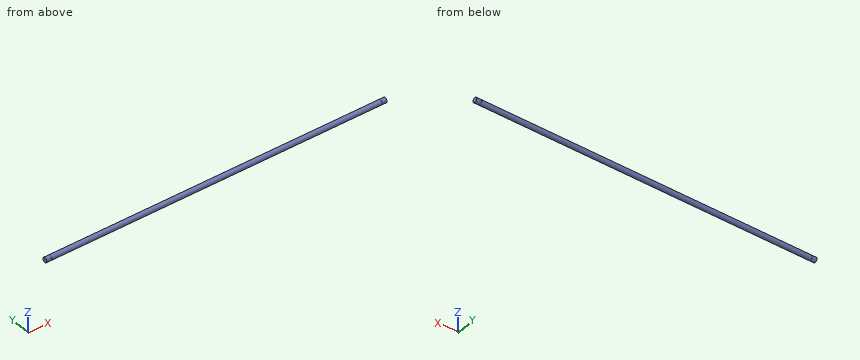
```python
from build123d import *

# Parameters (mm, degrees)
F0_R     = 5
F1_DEPTH = 350
F2_W     = 1.1
F2_H     = 1


with BuildPart() as f1:
    # F0 (on Right) → F1 (new body, symmetric)
    with BuildSketch(Plane.YZ):
        Circle(F0_R)
    extrude(amount=F1_DEPTH, both=True)

    # F2 (on Front) → F3 (revolve, cut)
    with BuildSketch(Plane.XZ):
        with Locations((340.05, 5.3)):
            Rectangle(F2_W, F2_H)
        with Locations((-340.05, 5.3)):
            Rectangle(F2_W, F2_H)
    revolve(axis=Axis((186.2977445126, 0, 0), (1, 0, 0)), mode=Mode.SUBTRACT)


solid = f1.part
```
Design review of the part built by this model. Coordinates are the model's own, in mm. Coordinates: 2 decimals unless noted, no trailing zeros. Write each loop counter-clockwise with the first axis right and the second up, starting at its lowest first coordinate (ties: lowest second). Pieces come first, ordered by that corner, then holes.
1) To check wall thickness, follow L1, parallel to Z at x = 173, y = 0.5; L2, parallel to Z at x = 239.5, y = 1.25. State the ranges of each line that lie inside material, in increasing order.
2) Add section C-C (x = 162). Write out the cut boundary in (y, z).
3) Add section B-B (z = 2). Write out the cut boundary in (x, y), plus the area to 3 significant figures.
4) Insertion check: pin 1 (5 mm diameter, centred on x = -176, y = -3, fed in from +Z); pin 2 (2 mm diameter, centred on x = 165, z = -3, fed in from -Y); pin 3 (2 mm diameter, centred on x = 207, y = 2.5, fed in from -Z). Each pin has a flat end and moves straight along its axis. Give the tip position at first contact, or say it passes through.
5) Add section A-A (y = -1.5). Write out the cut boundary in (x, z).
Check result:
1. L1: z = -4.97 to 4.97
1. L2: z = -4.84 to 4.84
2. outline: circle Ø10 at (0, 0)
3. outline: (-350, -4.58) - (-340.6, -4.58) - (-340.6, -4.36) - (-339.5, -4.36) - (-339.5, -4.58) - (339.5, -4.58) - (339.5, -4.36) - (340.6, -4.36) - (340.6, -4.58) - (350, -4.58) - (350, 4.58) - (340.6, 4.58) - (340.6, 4.36) - (339.5, 4.36) - (339.5, 4.58) - (-339.5, 4.58) - (-339.5, 4.36) - (-340.6, 4.36) - (-340.6, 4.58) - (-350, 4.58) - close
3. area: 6,410 mm2
4. pin 1: stops at z = 4.97
4. pin 2: stops at y = -4.58
4. pin 3: stops at z = -4.77
5. outline: (-350, -4.77) - (-340.6, -4.77) - (-340.6, -4.56) - (-339.5, -4.56) - (-339.5, -4.77) - (339.5, -4.77) - (339.5, -4.56) - (340.6, -4.56) - (340.6, -4.77) - (350, -4.77) - (350, 4.77) - (340.6, 4.77) - (340.6, 4.56) - (339.5, 4.56) - (339.5, 4.77) - (-339.5, 4.77) - (-339.5, 4.56) - (-340.6, 4.56) - (-340.6, 4.77) - (-350, 4.77) - close
